Input: dimensioned drawing with shaded views. Units: mm. Origin: part minimum x, y, z. Round coordinates to 2 decimals unless told otherwise and drop trailing zeros. Loops run counter-clockwise (first coordinate to the right, second up) from the corner with the lowest first, then second, coordinate; pieces in that order, holes last. Notation, with made-up numbers: (80, -36.75) - (106, -36.75) arc R7 cw to (106, -32.75) - close; hole circle Ø3 at (79, 64.5). An arc over 180 degrees is marked (long way). Answer as CSV lines item,"result".
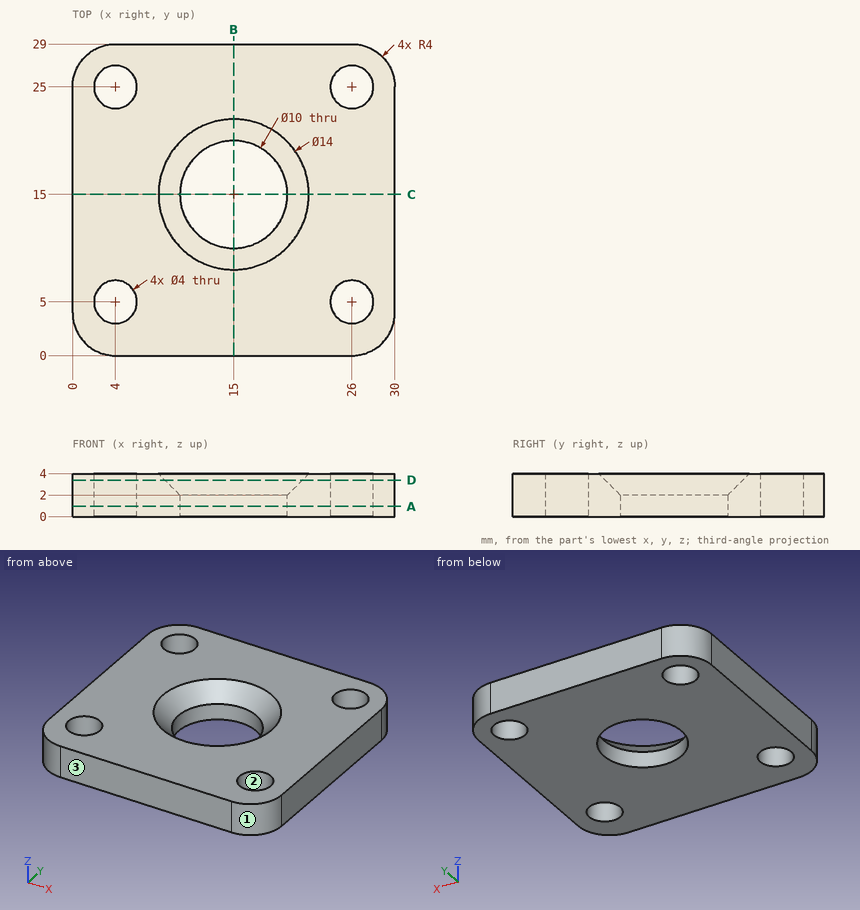
(1) Material intervals for line 1 along Y through (x, z) = (26, 2.1); line 2 along Y through (x, z) = (15, 0.5); line 3 along X through (y, z) = (4.5, 0.3), sorted ascending.
Findings below:
line 1,"0 to 3, 7 to 23, 27 to 29"
line 2,"0 to 10, 20 to 29"
line 3,"0 to 2.06, 5.94 to 24.06, 27.94 to 30"
(2) Section B-B (x = 15). Output: boundary loops of the cut face in (y, z), and give its area (3 significant figures).
Findings below:
outline,"(0, 0) - (10, 0) - (10, 2) - (8, 4) - (0, 4) - close; (20, 0) - (29, 0) - (29, 4) - (22, 4) - (20, 2) - close"
area,"72.0 mm2"
(3) Draft query along X for the marked faces 1, 2 and 3. Return one class per face: pulls with the +X half, pulls with the -X half, needs draft (parallel to the pull), parting line crosses it, or undercut.
Findings below:
face 1,"pulls with the +X half"
face 2,"undercut"
face 3,"needs draft"
(4) Section A-A (z = 0.95). Output: boundary loops of the cut face in (x, y), and give its area (3 significant figures).
Findings below:
outline,"(0, 4) arc R4 ccw to (4, 0) - (26, 0) arc R4 ccw to (30, 4) - (30, 25) arc R4 ccw to (26, 29) - (4, 29) arc R4 ccw to (0, 25) - close; hole circle Ø4 at (4, 5); hole circle Ø4 at (4, 25); hole circle Ø10 at (15, 15); hole circle Ø4 at (26, 5); hole circle Ø4 at (26, 25)"
area,"727 mm2"
(5) Section D-D (z = 3.4). Output: boundary loops of the cut face in (x, y), and give its area (3 significant figures).
Findings below:
outline,"(0, 4) arc R4 ccw to (4, 0) - (26, 0) arc R4 ccw to (30, 4) - (30, 25) arc R4 ccw to (26, 29) - (4, 29) arc R4 ccw to (0, 25) - close; hole circle Ø4 at (4, 5); hole circle Ø4 at (4, 25); hole circle Ø12.8 at (15, 15); hole circle Ø4 at (26, 5); hole circle Ø4 at (26, 25)"
area,"677 mm2"
(6) Section C-C (y = 15). Output: boundary loops of the cut face in (x, z).
Findings below:
outline,"(0, 0) - (10, 0) - (10, 2) - (8, 4) - (0, 4) - close; (20, 0) - (30, 0) - (30, 4) - (22, 4) - (20, 2) - close"
(7) Pin query (flat end, axial travel): P1, Ø3.5, axis at x = 26, y = 5, coming from the +Z side. Return the tip coordinate at first contact, or that it passes through.
Findings below:
P1,"through"
